Drawing for the job (mm, zero at the part's lowest x, y, z). Give positions to 0.01 mm unless a question says otherwise; leave off trailing zeros. Order: outer loops, then holes, each group sorted by start corner. A loop starts at its lowest first (then second) coordinate and runs counter-clockwise, first axis right, second up. Notation, with made-up numbers: (-6.5, -30) -> (10.5, -30) arc R14 ccw to (10.5, -15) -> close; hole circle Ø6 at (-10.5, 83.5). An arc over 180 degrees is marked (long way). Use one line per item in the form item = value. Start each with the question number.
1) Probe line 1 (Y direction, x = 20, z = 3.75); line 2 (X direction, y = 5.75, z = 5.25) (1 decimal); line 3 (X direction, y = 2.5, z = 0.5). List the from-to ranges inside material, lowest first.
2) Cut at B-B, the plane x = 20. Give the cut face in (y, z).
3) Cut at A-A, the plane y = 7.5. Give the cut face in (x, z).
4) Drop flat-ended pins along their axis: P1, Ø3, axis at x = 212.67, y = 7.5, coming from the -Z side; P2, Ø6, axis at x = 20, y = 7.5, coming from the +Z side; P3, Ø1, axis at y = 13, z = 0.5, coming from the +X side. Give the stop position or say it passes through.
5) Cut at C-C, the plane z = 5. Give the cut face in (x, y), and give its area (3 significant figures).
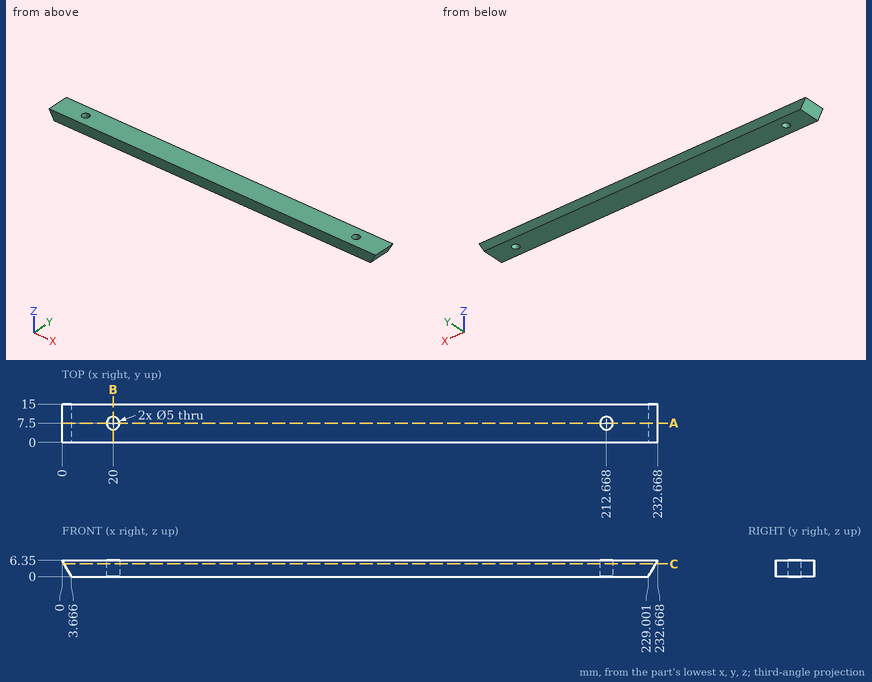
Result:
q1.line_1 = 0 to 5, 10 to 15
q1.line_2 = 0.6 to 18.2, 21.8 to 210.9, 214.5 to 232
q1.line_3 = 3.38 to 229.29
q2.outline = (0, 0) -> (5, 0) -> (5, 6.35) -> (0, 6.35) -> close; (10, 0) -> (15, 0) -> (15, 6.35) -> (10, 6.35) -> close
q3.outline = (0, 6.35) -> (3.67, 0) -> (17.5, 0) -> (17.5, 6.35) -> close; (22.5, 0) -> (210.17, 0) -> (210.17, 6.35) -> (22.5, 6.35) -> close; (215.17, 0) -> (229, 0) -> (232.67, 6.35) -> (215.17, 6.35) -> close
q4.P1 = through
q4.P2 = 6.35
q4.P3 = 229.58
q5.outline = (0.78, 0) -> (231.89, 0) -> (231.89, 15) -> (0.78, 15) -> close; hole circle Ø5 at (20, 7.5); hole circle Ø5 at (212.67, 7.5)
q5.area = 3,430 mm²
